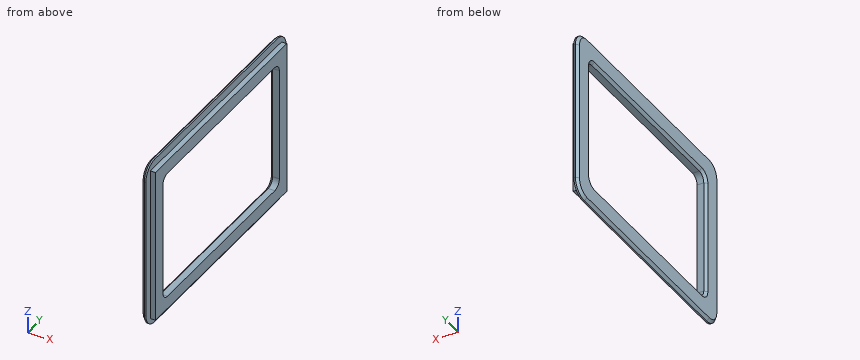
from build123d import *

# Parameters (mm, degrees)
SKETCH_W     = 440
SKETCH_H     = 300
PAD_DEPTH    = 10
PAD001_DEPTH = 8
CHAMFER_SIZE = 5


with BuildPart() as part:
    # Sketch → Pad (new body)
    with BuildSketch(Plane.YZ):
        Rectangle(SKETCH_W, SKETCH_H)
        with BuildLine():
            Line((-195, 110), (-195, -110))
            ThreePointArc((-195, -110), (-190.606602, -120.606602), (-180, -125))
            Line((-180, -125), (180, -125))
            ThreePointArc((180, -125), (190.606602, -120.606602), (195, -110))
            Line((195, -110), (195, 110))
            ThreePointArc((195, 110), (190.606602, 120.606602), (180, 125))
            Line((180, 125), (-180, 125))
            ThreePointArc((-180, 125), (-190.606602, 120.606602), (-195, 110))
        make_face(mode=Mode.SUBTRACT)
    extrude(amount=PAD_DEPTH)

    # Sketch001 (on Face13 of Pad) → Pad001 (join)
    with BuildSketch(Plane(origin=(0, 0, 0), x_dir=(0, 1, 0), z_dir=(-1, 0, 0))):
        with BuildLine():
            Line((-235, 135), (-235, -135))
            ThreePointArc((-235, -135), (-226.213203, -156.213203), (-205, -165))
            Line((-205, -165), (205, -165))
            ThreePointArc((205, -165), (226.213203, -156.213203), (235, -135))
            Line((235, -135), (235, 135))
            ThreePointArc((235, 135), (226.213203, 156.213203), (205, 165))
            Line((205, 165), (-205, 165))
            ThreePointArc((-205, 165), (-226.213203, 156.213203), (-235, 135))
        make_face()
        with BuildLine():
            Line((-195, 110), (-195, -110))
            ThreePointArc((-195, -110), (-190.606602, -120.606602), (-180, -125))
            Line((-180, -125), (180, -125))
            ThreePointArc((180, -125), (190.606602, -120.606602), (195, -110))
            Line((195, -110), (195, 110))
            ThreePointArc((195, 110), (190.606602, 120.606602), (180, 125))
            Line((180, 125), (-180, 125))
            ThreePointArc((-180, 125), (-190.606602, 120.606602), (-195, 110))
        make_face(mode=Mode.SUBTRACT)
    extrude(amount=PAD001_DEPTH)

    # Chamfer
    chamfer_edges = [part.edges().sort_by_distance(p)[0] for p in [
        (-8, -235, 0),
        (-8, -226.213203, 156.213203),
        (-8, 0, 165),
        (-8, 226.213203, 156.213203),
        (-8, 235, 0),
        (-8, 226.213203, -156.213203),
        (-8, 0, -165),
        (-8, -226.213203, -156.213203),
        (-8, -195, 0),
        (-8, -190.606602, 120.606602),
        (-8, 0, 125),
        (-8, 190.606602, 120.606602),
        (-8, 195, 0),
        (-8, 190.606602, -120.606602),
        (-8, 0, -125),
        (-8, -190.606602, -120.606602),
    ]]
    chamfer(chamfer_edges, length=CHAMFER_SIZE)


solid = part.part
Part model, mm, in its own coordinate system. Round coordinates to 2 decimals unless told otherwise and drop trailing zeros. Write each loop counter-clockwise with the first axis right and the second up, starting at its lowest first coordinate (ties: lowest second). Pieces come first, ordered by that corner, then holes. Notation, with made-up numbers: M -29,80 L 0,80 A13 cw 0,89 Z; hole C 68,18 d3. An arc over 180 degrees is marked long. Return JSON: item names as keys, results as strings. Group by question number.
(1) Saw through at C-C on y = -43. Write the cut outline in (x, z).
(2) Drill centre lines: probe 1 along Y at (x, z) = (6.5, -110); probe 2 along Z at (x, y) = (7.5, 23.5); probe 3 along Z at (x, y) = (-1, 90). Where is each one in solid material? Low to high.
(3) Pin check, flat tips, straight feed: pin 1 Ø6 at (x, z) = (-4.5, 96.5) entering from +Y; pin 2 Ø4 at (x, y) = (2.5, -59.5) entering from +Z; pin 3 Ø5 at (x, z) = (7, 42) entering from -Y; pin 4 Ø5 at (x, z) = (3, 65) entering from +Y. Stop position of each tip, or through.
(4) Saw through at B-B on x = 6.5. Write the cut outline in (y, z), then the cut area to 3 significant figures.
(5) Saw through at A-A on z = 50. Write the cut outline in (x, y), then the cut area to 3 significant figures.
Returned:
{
 "1": {"outline": "M -8,-160 L -3,-165 L 0,-165 L 0,-150 L 10,-150 L 10,-125 L -3,-125 L -8,-130 Z; M -8,130 L -3,125 L 10,125 L 10,150 L 0,150 L 0,165 L -3,165 L -8,160 Z"},
 "2": {"probe 1": "-220 to -195, 195 to 220", "probe 2": "-150 to -125, 125 to 150", "probe 3": "-165 to -125, 125 to 165"},
 "3": {"pin 1": "y = 235", "pin 2": "z = 150", "pin 3": "y = -220", "pin 4": "y = 220"},
 "4": {"outline": "M -220,-150 L 220,-150 L 220,150 L -220,150 Z; hole M -195,-110 A15 ccw -180,-125 L 180,-125 A15 ccw 195,-110 L 195,110 A15 ccw 180,125 L -180,125 A15 ccw -195,110 Z", "area": "34,700 mm²"},
 "5": {"outline": "M -8,-230 L -3,-235 L 0,-235 L 0,-220 L 10,-220 L 10,-195 L -3,-195 L -8,-200 Z; M -8,200 L -3,195 L 10,195 L 10,220 L 0,220 L 0,235 L -3,235 L -8,230 Z", "area": "1,090 mm²"}
}
